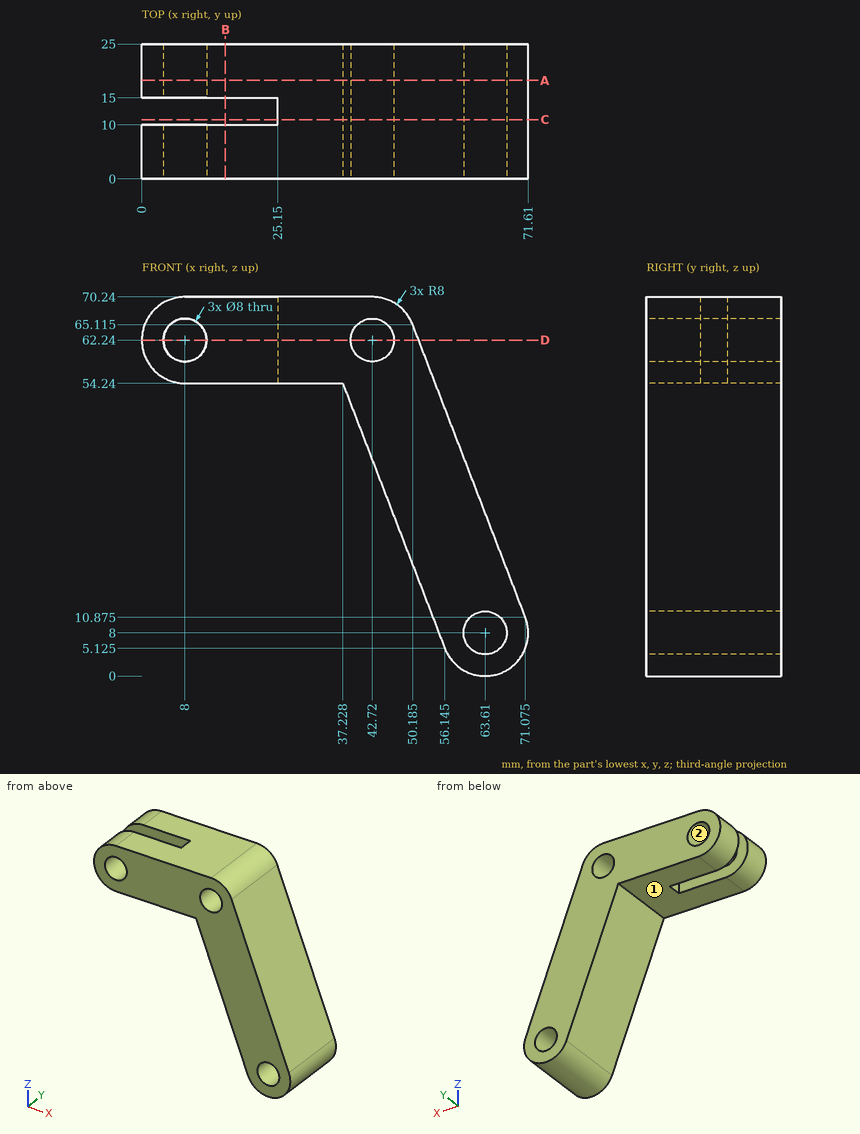
Can you work these out from the drawing? Everything is in mm from the part's minimum corner. A direction names the side the tool comes from. Round coordinates to 2 decimals unless told otherwise and drop trailing zeros. Write each loop counter-clockwise with the first axis right and the second up, starting at its lowest first coordinate (ties: lowest second). Pieces come first, ordered by that corner, then holes. Notation, with made-up numbers: (15, -2) - (55, -2) arc R17 ccw to (55, 17) - close; hole circle Ø8 at (-21, -28). An arc over 180 degrees is marked (long way). Put each result on its own line as item: value. Start each with the question number.
(1) Will these pins go through, and if not, where does the flat tip stop? pin 1 (4 mm diameter, centred on y = 13.5, z = 60, fed in from -X); pin 2 (4 mm diameter, centred on x = 34, y = 16, fed in from -Z); pin 3 (3 mm diameter, centred on y = 10.5, z = 35.5, fed in from +X).
(2) I want a section at C-C, the plane y = 11. Give the number of separate pieces and of enclosed holes in the cut face, plus the area to 3 significant figures.
(3) I want a section at D-D, the plane z = 62.24. Please give me the cut outline in (x, y).
(4) I want a section at B-B, the plane x = 15.5. Please give me the cut outline in (y, z), plus the area to 3 significant figures.
(5) For the marked faces 1 and 2, which set-ups out of +Z, -Z, +X, -X, +Y, -Y let a thin tool reach every point of the face, with its end or its side?
(6) I need wall thicknesses on probe 1 along Z at (x, y) = (8, 5.25); probe 2 along X at (y, z) = (7.75, 62.24); probe 3 along X at (y, z) = (23.25, 63) (1 decimal). Which ranges of each line are inside material? Lowest first, please.
(7) I want a section at A-A, the plane y = 18.25. Please give me the cut outline in (x, z) (1 decimal), plus the area to 3 significant figures.
Here are the results:
1. pin 1: stops at x = 0.05
1. pin 2: stops at z = 54.24
1. pin 3: stops at x = 62.17
2. separate pieces: 1
2. enclosed holes: 2
2. area: 1,210 mm^2
3. outline: (0, 0) - (4, 0) - (4, 10) - (0, 10) - close; (0, 15) - (4, 15) - (4, 25) - (0, 25) - close; (12, 0) - (38.72, 0) - (38.72, 25) - (12, 25) - (12, 15) - (25.15, 15) - (25.15, 10) - (12, 10) - close; (46.72, 0) - (51.29, 0) - (51.29, 25) - (46.72, 25) - close
4. outline: (0, 54.24) - (10, 54.24) - (10, 70.24) - (0, 70.24) - close; (15, 54.24) - (25, 54.24) - (25, 70.24) - (15, 70.24) - close
4. area: 320 mm^2
5. face 1: -Z, -X, +Y, -Y
5. face 2: +Y, -Y
6. probe 1: z = 54.24 to 58.24, 66.24 to 70.24
6. probe 2: x = 0 to 4, 12 to 38.72, 46.72 to 51.29
6. probe 3: x = 0 to 4.1, 11.9 to 38.8, 46.6 to 51
7. outline: (8, 54.2) - (37.2, 54.2) - (56.1, 5.1) arc R8 ccw to (71.1, 10.9) - (50.2, 65.1) arc R8 ccw to (42.7, 70.2) - (8, 70.2) arc R8 ccw to start; hole circle Ø8 at (8, 62.2); hole circle Ø8 at (42.7, 62.2); hole circle Ø8 at (63.6, 8)
7. area: 1,530 mm^2
